Read the model definition and answer for the solid it produces. Units are mm, in the model's axes. Coordinates: 2 decimals unless noted, no trailing zeros. Loops run counter-clockwise (first coordinate to the right, second up) from the corner with the lowest first, then second, coordinate; pieces in that order, holes last.
from build123d import *

# Parameters (mm, degrees)
F1_DEPTH = 10
F2_R     = 5


with BuildPart() as f1:
    # F0 (on Front) → F1 (new body)
    with BuildSketch(Plane.XZ):
        with BuildLine():
            ThreePointArc((0, 50), (35.355339, 35.355339), (50, 0))
            Line((50, 0), (55, 0))
            ThreePointArc((55, 0), (38.890873, 38.890873), (0, 55))
            Line((0, 55), (0, 50))
        make_face()
    extrude(amount=F1_DEPTH)

    # F2
    f2_edges = [f1.edges().sort_by_distance(p)[0] for p in [
        (50, -5, 0),
        (0, -5, 50),
    ]]
    fillet(f2_edges, radius=F2_R)


solid = f1.part
Item 1: Find the intervals of material crossed by line 1 along Z through (x, y) = (18.5, -3.75); line 2 along Z through (x, y) = (10, -5.25); line 3 along X through (y, z) = (-5, 35), in increasing order.
Numbers:
line 1: z = 46.45 to 51.8
line 2: z = 48.99 to 54.08
line 3: x = 35.71 to 42.43
Item 2: A cutting plane is placed at B-B on x = 10. Determine the outline of the cut face in (y, z).
Numbers:
outline: (-10, 48.99) - (0, 48.99) - (0, 54.08) - (-10, 54.08) - close
Item 3: A cutting plane is placed at C-C on z = 9.5. Determine the outline of the cut face in (x, y).
Numbers:
outline: (49.09, -10) - (54.17, -10) - (54.17, 0) - (49.09, 0) - close
Item 4: A cutting plane is placed at A-A on y = -1. Determine the outline of the cut face in (x, z).
Numbers:
outline: (0, 54.77) arc R5 ccw to (4.55, 49.79) arc R50 cw to (49.79, 4.55) arc R5 ccw to (54.77, 0) - (55, 0) arc R55 ccw to (0, 55) - close
Item 5: Given pin 1 (6 mm diameter, centred on x = 42, y = -7.5, fed in from +Z); pin 2 (2 mm diameter, centred on y = -7, z = 9, fed in from +X); pin 3 (4 mm diameter, centred on x = 19, y = -5.5, fed in from -Z), each flat-ended and moving along its own axis, determine where each tip first touches the part or whether it passes through.
Numbers:
pin 1: stops at z = 38.78
pin 2: stops at x = 54.42
pin 3: stops at z = 45.38
